Input: part model. Units: mm. Frame: model coordinates. Coordinates: 2 decimals unless noted, no trailing zeros. Order: outer loops, then holes, each group sorted by start corner. A loop starts at its lowest first (then second) coordinate and runs counter-clockwise, first axis right, second up. Notation, with made-up numbers: (-33, 43.25) -> (6, 43.25) arc R26 cw to (6, 74.25) -> close; hole circle Ø10 at (31.5, 45). An arc over 180 degrees is marked (long way). Use one line per item in the form item = value. Start each with the question number.
1) Draft query along Y for faces 1 (the cylindrical face through (14.386, -16.172, 1.568)), 2 (the flat face through (-1, 1, 0)). Return one class per face: pulls with the +Y half, pulls with the -Y half, needs draft (parallel to the pull), parting line crosses it, or undercut.
2) Pin query (flat end, axial travel): pin 1 (1.6 mm diameter, centred on x = -63, z = 2.5, fed in from +Y); pin 2 (1 mm diameter, centred on x = -88.5, z = 2, fed in from -Y) (3 decimals); pin 3 (1.6 mm diameter, centred on x = -88, z = 1.5, fed in from +Y) (3 decimals). Return the tip coordinate at first contact, or that it passes through.
3) Ray query, line 1 along X through (y, z) = (-13, 1.95); line 2 along X through (y, z) = (-20, 2.75); line 3 along Y through (x, z) = (-1, 0.7). Return the intervals inside material, ascending.
4) Section query A-A on z = 0.55. Output: boundary loops of the cut face in (x, y) (3 decimals), then the cut area to 3 significant figures.
5) Section query B-B on y = -35.5. Output: boundary loops of the cut face in (x, z), then the cut area to 3 significant figures.
from build123d import *

# Parameters (mm, degrees)
SKETCH3_W           = 180
SKETCH3_H           = 180
SKETCH3_R           = 8.616960002
SKETCH3_R_2         = 8.643887018
SKETCH3_R_3         = 1.43602308
SKETCH3_R_4         = 1.4
SKETCH3_R_5         = 1.467212263
BOSS_EXTRUDE1_DEPTH = 3.18
SKETCH4_W           = 80
SKETCH4_H           = 3.18
CUT_EXTRUDE1_DEPTH  = 128.318939675
SKETCH5_W           = 3.18
SKETCH5_H           = 80.125
CUT_EXTRUDE2_DEPTH  = 128.318939675


with BuildPart() as part:
    # Sketch3 → Boss-Extrude1 (new body)
    with BuildSketch(Plane.XY):
        Rectangle(SKETCH3_W, SKETCH3_H)
        with Locations(Location((-3.22889268, -13.57556396, 0), (0, 0, 180))):
            Circle(SKETCH3_R, mode=Mode.SUBTRACT)
        with Locations(Location((22.63110732, -13.57556396, 0), (0, 0, 180))):
            Circle(SKETCH3_R_2, mode=Mode.SUBTRACT)
        with Locations(Location((0, -88, 0), (0, 0, 180))):
            Circle(SKETCH3_R_3, mode=Mode.SUBTRACT)
        with Locations(Location((0.844873764, 43.606084924, 0), (0, 0, 180))):
            Circle(SKETCH3_R_4, mode=Mode.SUBTRACT)
        with Locations(Location((14.594873764, 65.106084924, 0), (0, 0, 180))):
            Circle(SKETCH3_R_4, mode=Mode.SUBTRACT)
        with Locations(Location((28.344873764, 43.606084924, 0), (0, 0, 180))):
            Circle(SKETCH3_R_5, mode=Mode.SUBTRACT)
    extrude(amount=BOSS_EXTRUDE1_DEPTH)

    # Sketch4 → Cut-Extrude1 (cut, through all)
    with BuildSketch(Plane.XY.offset(3.18)):
        with Locations((50, -88.41)):
            Rectangle(SKETCH4_W, SKETCH4_H)
        with Locations((-50, 88.41)):
            Rectangle(SKETCH4_W, SKETCH4_H)
        with Locations((50, 88.41)):
            Rectangle(SKETCH4_W, SKETCH4_H)
        with Locations((-50, -88.41)):
            Rectangle(SKETCH4_W, SKETCH4_H)
    extrude(amount=-CUT_EXTRUDE1_DEPTH, mode=Mode.SUBTRACT)

    # Sketch5 → Cut-Extrude2 (cut, through all)
    with BuildSketch(Plane.XY.offset(3.18)):
        with Locations((-88.41, 49.9375)):
            Rectangle(SKETCH5_W, SKETCH5_H)
        with Locations((-88.41, -49.9375)):
            Rectangle(SKETCH5_W, SKETCH5_H)
        with Locations((88.41, -49.9375)):
            Rectangle(SKETCH5_W, SKETCH5_H)
        with Locations((88.41, 49.9375)):
            Rectangle(SKETCH5_W, SKETCH5_H)
    extrude(amount=-CUT_EXTRUDE2_DEPTH, mode=Mode.SUBTRACT)


solid = part.part
Answers below:
q1.face_1 = undercut
q1.face_2 = needs draft
q2.pin_1 = 86.82
q2.pin_2 = -9.875
q2.pin_3 = 9.875
q3.line_1 = -86.82 to -11.83, 5.37 to 14.01, 31.26 to 86.82
q3.line_2 = -86.82 to -8.97, 2.51 to 16.85, 28.41 to 86.82
q3.line_3 = -90 to -89.03, -86.97 to -21.9, -5.25 to 90
q4.outline = (-90, -9.875) -> (-86.82, -9.875) -> (-86.82, -86.82) -> (-10, -86.82) -> (-10, -90) -> (10, -90) -> (10, -86.82) -> (86.82, -86.82) -> (86.82, -9.875) -> (90, -9.875) -> (90, 9.875) -> (86.82, 9.875) -> (86.82, 86.82) -> (10, 86.82) -> (10, 90) -> (-10, 90) -> (-10, 86.82) -> (-86.82, 86.82) -> (-86.82, 9.875) -> (-90, 9.875) -> close; hole circle Ø17.234 at (-3.229, -13.576); hole circle Ø2.872 at (0, -88); hole circle Ø2.8 at (0.845, 43.606); hole circle Ø2.8 at (14.595, 65.106); hole circle Ø17.288 at (22.631, -13.576); hole circle Ø2.934 at (28.345, 43.606)
q4.area = 29,900 mm^2
q5.outline = (-86.82, 0) -> (86.82, 0) -> (86.82, 3.18) -> (-86.82, 3.18) -> close
q5.area = 552 mm^2
